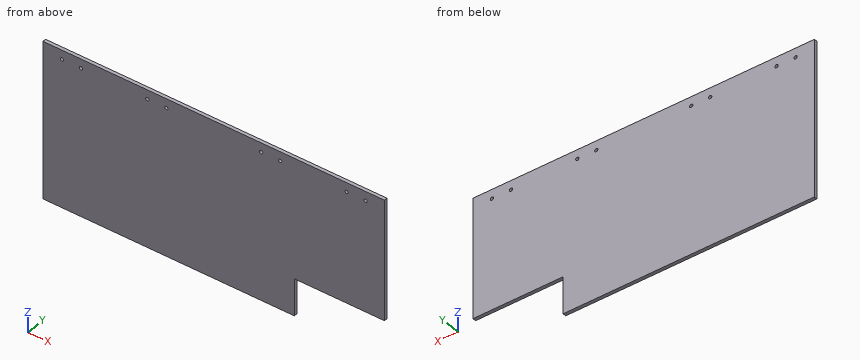
```python
from build123d import *

# Parameters (mm, degrees)
SKETCH1_W           = 360
SKETCH1_H           = 170
BOSS_EXTRUDE1_DEPTH = 3.5
SKETCH2_R           = 1.75
CUT_EXTRUDE1_DEPTH  = 3.5
CUT_EXTRUDE2_REACH  = 5.5
SKETCH3_W           = 95
SKETCH3_H           = 40


with BuildPart() as part:
    # Sketch1 → Boss-Extrude1 (new body)
    with BuildSketch(Plane(origin=(0, 0, 0), x_dir=(1, 0, 0), z_dir=(0, 1, 0))):
        with Locations((180, 85)):
            Rectangle(SKETCH1_W, SKETCH1_H)
    extrude(amount=BOSS_EXTRUDE1_DEPTH)

    # Sketch2 → Cut-Extrude1 (cut)
    with BuildSketch(Plane(origin=(0, 3.5, 0), x_dir=(1, 0, 0), z_dir=(0, 1, 0))):
        with Locations((20, 10)):
            Circle(SKETCH2_R)
        with Locations((40, 10)):
            Circle(SKETCH2_R)
        with Locations((110, 10)):
            Circle(SKETCH2_R)
        with Locations((130, 10)):
            Circle(SKETCH2_R)
        with Locations((230, 10)):
            Circle(SKETCH2_R)
        with Locations((250, 10)):
            Circle(SKETCH2_R)
        with Locations((320, 10)):
            Circle(SKETCH2_R)
        with Locations((340, 10)):
            Circle(SKETCH2_R)
    extrude(amount=-CUT_EXTRUDE1_DEPTH, mode=Mode.SUBTRACT)

    # Sketch3 → Cut-Extrude2 (cut, up to next)
    with BuildSketch(Plane(origin=(0, 3.5, 0), x_dir=(1, 0, 0), z_dir=(0, 1, 0)), mode=Mode.PRIVATE) as cut_extrude2_sk1:
        with Locations((312.5, 150)):
            Rectangle(SKETCH3_W, SKETCH3_H)
    cut_extrude2_tool1 = extrude(cut_extrude2_sk1.sketch, amount=-CUT_EXTRUDE2_REACH, mode=Mode.PRIVATE) & part.part
    add(cut_extrude2_tool1.solids().sort_by_distance((312.5, 3.5, -150))[0], mode=Mode.SUBTRACT)


solid = part.part
```
Here's how the part is built. I have some questions about the finished solid (model axes, mm). Round coordinates to 2 decimals unless told otherwise and drop trailing zeros. Loops run counter-clockwise (first coordinate to the right, second up) from the corner with the lowest first, then second, coordinate; pieces in that order, holes last.
1. Will this pin go through, and if not, where does the flat tip stop? pin 1 (3 mm diameter, centred on x = 110, z = -10, fed in from +Y).
Answers:
pin 1: passes through
2. Suppose I cut it at B-B, the plane z = -158.5. Please give me the cut outline in (x, y), and give its area (4 significant figures).
Answers:
outline: (0, 0) - (265, 0) - (265, 3.5) - (0, 3.5) - close
area: 927.5 mm2
3. Suppose I cut it at A-A, the plane y = 1.1. Give the number of separate pieces and of enclosed holes in the cut face, and give its area (3 significant figures).
Answers:
separate pieces: 1
enclosed holes: 8
area: 57,300 mm2
4. If I drill on probe 1 along Z at (x, y) = (110, 2.75); probe 2 along Z at (x, y) = (310, 0.75); probe 3 along X at (y, z) = (1.3, -163), over which ranges is the centre line in solid material (lowest first)?
Answers:
probe 1: z = -170 to -11.75, -8.25 to 0
probe 2: z = -130 to 0
probe 3: x = 0 to 265
